Part print with two shaded views. Sizes in mm from the minimum x, y, z corner. Give positions to 0.01 mm unless a question says otherwise; leave off trailing zeros. Loops run counter-clockwise (first coordinate to the right, second up) from the corner with the lowest first, then second, coordinate; pieces in that order, holes last. Notation, with made-up numbers: M 26,-37.75 L 49,-37.75 A18 ccw 49,-4.75 Z; hole C 70,24.5 d1. An arc over 180 degrees is marked long. Answer in a Markdown table with one row per item.
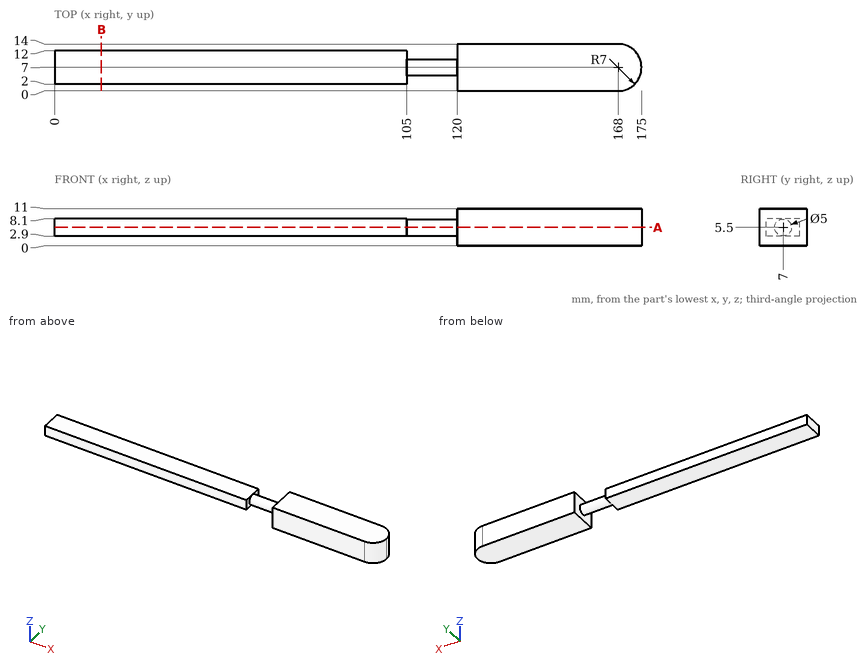
Q1. Saw through at A-A (z = 5.5). Give the cut face in (x, y).
Reported:
| item | result |
|---|---|
| outline | M 0,2 L 105,2 L 105,4.5 L 120,4.5 L 120,0 L 168,0 A7 ccw 175,7 A7 ccw 168,14 L 120,14 L 120,9.5 L 105,9.5 L 105,12 L 0,12 Z |
Q2. Drop flat-ended pins along their axis: pin 1 (4 mm diameter, centred on x = 114.5, z = 7, fed in from +Y); pin 2 (3.5 mm diameter, centred on y = 9.5, z = 6, fed in from -X); pin 3 (5.5 mm diameter, centred on x = 68.5, z = 4.5, fed in from +Y); pin 4 (2 mm diameter, centred on y = 4, z = 9.5, fed in from +X). Give the stop position or say it passes through.
Reported:
| item | result |
|---|---|
| pin 1 | y = 9.5 |
| pin 2 | x = 0 |
| pin 3 | y = 12 |
| pin 4 | x = 174.71 |
Q3. Saw through at B-B (x = 14). Give the cut face in (y, z).
Reported:
| item | result |
|---|---|
| outline | M 2,2.9 L 12,2.9 L 12,8.1 L 2,8.1 Z |
Q4. Probe probe 1 along Z at (x, y) = (94, 8); probe 2 along Y at (x, z) = (77, 8); probe 3 along X at (y, z) = (6.5, 3.5). List the from-to ranges inside material, lowest first.
Reported:
| item | result |
|---|---|
| probe 1 | 2.9 to 8.1 |
| probe 2 | 2 to 12 |
| probe 3 | 0 to 174.98 |
